Drawing for the job (mm, zero at the part's lowest x, y, z). Round coordinates to 2 decimals unless told otherwise and drop trailing zeros. Write each loop counter-clockwise with the first axis right and the second up, starting at its lowest first coordinate (ties: lowest second). Pieces come first, ordered by that corner, then holes. Notation, with made-up numbers: (20, 55.25) -> (46, 55.25) arc R26 cw to (46, 78.25) -> close; hole circle Ø2 at (-29.75, 15.5). An arc over 180 degrees is marked (long way). One line per question, with ' | ' between items.
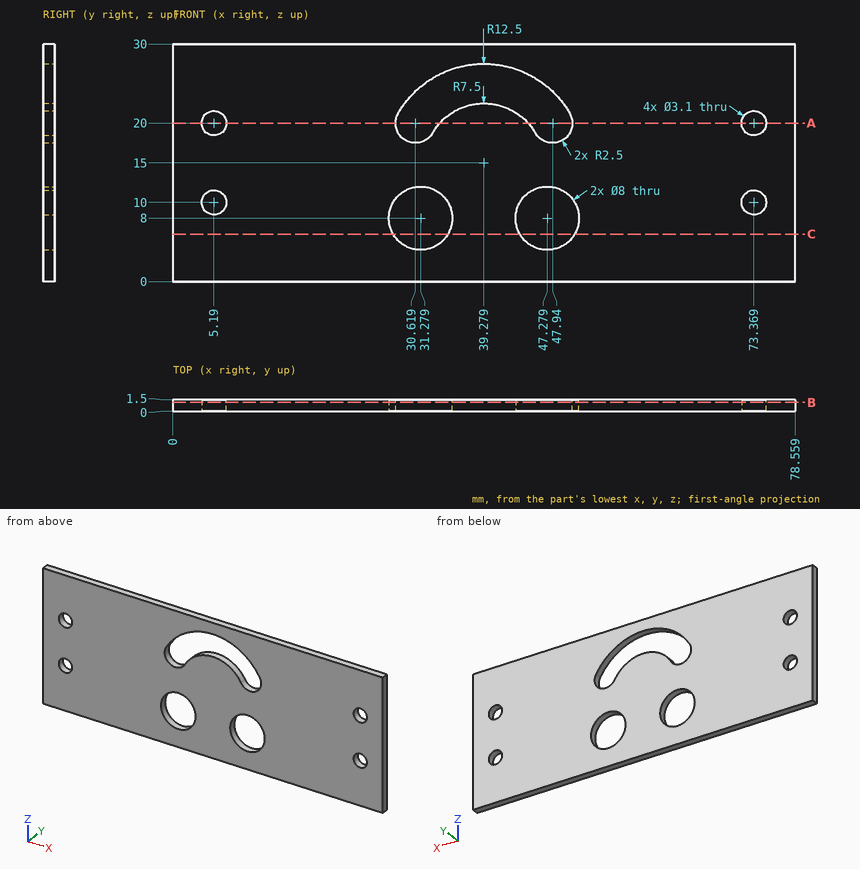
(1) Slice it at C-C (z = 6). Write the cut outline in (x, y) (1 decimal).
Calculated:
outline: (0, 0) -> (27.8, 0) -> (27.8, 1.5) -> (0, 1.5) -> close; (34.7, 0) -> (43.8, 0) -> (43.8, 1.5) -> (34.7, 1.5) -> close; (50.7, 0) -> (78.6, 0) -> (78.6, 1.5) -> (50.7, 1.5) -> close
(2) Slice it at A-A (z = 20). Write the cut outline in (x, y).
Calculated:
outline: (0, 0) -> (3.64, 0) -> (3.64, 1.5) -> (0, 1.5) -> close; (6.74, 0) -> (28.12, 0) -> (28.12, 1.5) -> (6.74, 1.5) -> close; (33.69, 0) -> (44.87, 0) -> (44.87, 1.5) -> (33.69, 1.5) -> close; (50.44, 0) -> (71.82, 0) -> (71.82, 1.5) -> (50.44, 1.5) -> close; (74.92, 0) -> (78.56, 0) -> (78.56, 1.5) -> (74.92, 1.5) -> close
(3) Drop a flat-ended pin along its axis: pin 1 (1.9 mm diameter, centred on x = 73.37, z = 10, fed in from -Y). Give the stop position or say it passes through.
Calculated:
pin 1: through
(4) Slice it at B-B (y = 1.15). State how many separate pieces and enclosed holes the cut face has, then the cut area to 3 significant figures.
Calculated:
separate pieces: 1 | enclosed holes: 7 | area: 2,100 mm2
(5) Wall check: line 1 (Z direction, x = 5.19, y = 0.55); line 2 (X direction, y = 0.95, z = 10.25) (1 decimal); line 3 (Z direction, x = 48, y = 0.8) (1 decimal). Give the ranges that are in metal, low to high. Write a range as from..to.
Calculated:
line 1: 0..8.45, 11.55..18.45, 21.55..30 | line 2: 0..3.7, 6.7..28, 34.6..44, 50.6..71.8, 74.9..78.6 | line 3: 0..4.1, 11.9..17.5, 24..30
